```python
from build123d import *

# Parameters (mm, degrees)
F1_DEPTH = 1.6
F3_DEPTH = 20
F5_DEPTH = 34.001
F6_W     = 34
F6_H     = 34
F6_W_2   = 30.5
F6_H_2   = 30.5
F7_DEPTH = 10
F6_R     = 8
F8_DEPTH = 16.7997198341


# Not quite as in the source:
# - a feature names something its author has since deleted; it is built from what else it names


with BuildPart() as f1:
    # F0 (on Top) → F1 (new body)
    with BuildSketch(Plane.XY):
        Polygon((-12.4, 19), (-17, 19), (-17, -19), (-12.4, -19), (-12.4, -20.5), (-5.9, -20.5), (-5.9, -19), (5.9, -19), (5.9, -20.5), (12.4, -20.5), (12.4, -19), (17, -19), (17, 19), (12.4, 19), (12.4, 20.5), (5.9, 20.5), (5.9, 19), (-5.9, 19), (-5.9, 20.5), (-12.4, 20.5), align=None)
    extrude(amount=F1_DEPTH)

    # F2 (on face) → F3 (join)
    with BuildSketch(Plane.XY.offset(1.6)):
        Polygon((-12.4, 19), (-17, 19), (-17, -19), (-12.4, -19), (-5.9, -19), (5.9, -19), (12.4, -19), (17, -19), (17, 19), (12.4, 19), (5.9, 19), (-5.9, 19), align=None)
    extrude(amount=F3_DEPTH)

    # F4 (on face) → F5 (cut, through all)
    with BuildSketch(Plane(origin=(-17, 0, 0), x_dir=(0, -1, 0), z_dir=(-1, 0, 0))):
        Polygon((-19, 17.3308689021), (19, 3.5), (19, 21.6), (-19, 21.6), align=None)
    extrude(amount=-F5_DEPTH, mode=Mode.SUBTRACT)

    # F6 (on face) → F7 (join)
    with BuildSketch(Plane(origin=(0, -3.3474561073, 9.1970600675), x_dir=(1, 0, 0), z_dir=(0, -0.3420201433, 0.9396926208))):
        with Locations((0, 4.0929107067)):
            Rectangle(F6_W, F6_H)
        with Locations((0, 4.0929107067)):
            Rectangle(F6_W_2, F6_H_2, mode=Mode.SUBTRACT)
    extrude(amount=F7_DEPTH)

    # F6 (on face) → F8 (cut, through all)
    with BuildSketch(Plane(origin=(0, -3.3474561073, 9.1970600675), x_dir=(1, 0, 0), z_dir=(0, -0.3420201433, 0.9396926208))):
        with Locations((0, 4.0929107067)):
            Circle(F6_R)
    extrude(amount=-F8_DEPTH, mode=Mode.SUBTRACT)


solid = f1.part
```
Model file for the job. Use its own axes, mm. A direction names the side the tool comes from. Give positions to 0.01 mm unless a question says otherwise; leave off trailing zeros. Write each loop counter-clockwise with the first axis right and the second up, starting at its lowest first coordinate (ties: lowest second). Pieces come first, ordered by that corner, then holes. Notation, with made-up numbers: (-10.5, -33) -> (6.5, -33) arc R20 cw to (6.5, -16) -> close; hole circle Ø3 at (-37.5, 80.25). An arc over 180 degrees is marked (long way). Use CSV: the item, a comma, the result in double quotes. Start each with the question number.
1) Pin check, flat tips, straight feed: P1, Ø0.8, axis at y = -19.5, z = 0.5, coming from the +X side; P2, Ø1, axis at x = -2.5, z = 1.5, coming from the -Y side; P3, Ø0.8, axis at y = 19.5, z = 1, coming from the -X side. Stop position of each tip, or through.
2) Two-plate mould, pull along X, no slides. Class faces 1 (the flat face through (-17, 0, 10)), 2 (the flat face through (6.6, 7.1, 13)), 3 (the flat face through (-4, -4, 0)): released by +X, released by -X, zero draft, split by the parting line, or undercut.
3) Tool access for faces 4 (the flat face through (5.9, 20, 1)), 5 (the flat face through (12.4, -20, 1)), 6 (the flat face through (5.9, -20, 1)), 7 (the flat face through (-9, -20, 1.6)): list every direction of +Z, -Z, +X, -X, +Y, -Y with a clear straight run to the whole face (end or side of a thin tool).
4) Drill centre lines: L1, parallel to X at y = 5, z = 22; L2, parallel to Y at x = -8.5, z = 2; L3, parallel to X at y = 10, z = 6. Where is each one in solid material? Low to high.
5) Cut at B-B on x = 13. List the corners of the cut face in (y, z), plus the area to 3 significant figures.
6) Cut at C-C on y = -11.5. List the corners of the cut face in (x, z), plus the area to 3 significant figures.
7) Cut at A-A on x = -4.5. List the corners of the cut face in (y, z), plus the area to 3 significant figures.
8) Cut at D-D on z = 21.5. List the corners of the cut face in (x, y), plus the area to 3 significant figures.
Final values:
1,P1,"stops at x = 12.4"
1,P2,"stops at y = -19"
1,P3,"stops at x = -12.4"
2,face 1,"released by -X"
2,face 2,"undercut"
2,face 3,"zero draft"
3,face 4,"+Z, -Z, +Y"
3,face 5,"+Z, -Z, +X, -Y"
3,face 6,"+Z, -Z, -Y"
3,face 7,"+Z, +X, -X, -Y"
4,L1,"x = -17 to -15.25, 15.25 to 17"
4,L2,"y = -19 to 19"
4,L3,"x = -17 to -3.14, 3.14 to 17"
5,outline,"(-19, 0) -> (19, 0) -> (19, 17.33) -> (16.47, 16.41) -> (13.05, 25.81) -> (11.41, 25.21) -> (14.83, 15.81) -> (-13.83, 5.38) -> (-17.25, 14.78) -> (-18.9, 14.18) -> (-15.48, 4.78) -> (-19, 3.5) -> close"
5,area,"431 mm2"
6,outline,"(-17, 0) -> (17, 0) -> (17, 16.87) -> (15.25, 16.87) -> (15.25, 6.23) -> (-15.25, 6.23) -> (-15.25, 16.87) -> (-17, 16.87) -> close"
6,area,"249 mm2"
7,outline,"(-19, 0) -> (-2.68, 0) -> (-5.72, 8.33) -> (-13.83, 5.38) -> (-17.25, 14.78) -> (-18.9, 14.18) -> (-15.48, 4.78) -> (-19, 3.5) -> close; (6.71, 12.86) -> (11.39, 0) -> (19, 0) -> (19, 17.33) -> (16.47, 16.41) -> (13.05, 25.81) -> (11.41, 25.21) -> (14.83, 15.81) -> close"
7,area,"282 mm2"
8,outline,"(-17, 1.22) -> (-15.25, 1.22) -> (-15.25, 12.76) -> (15.25, 12.76) -> (15.25, 1.22) -> (17, 1.22) -> (17, 14.62) -> (-17, 14.62) -> close"
8,area,"104 mm2"
